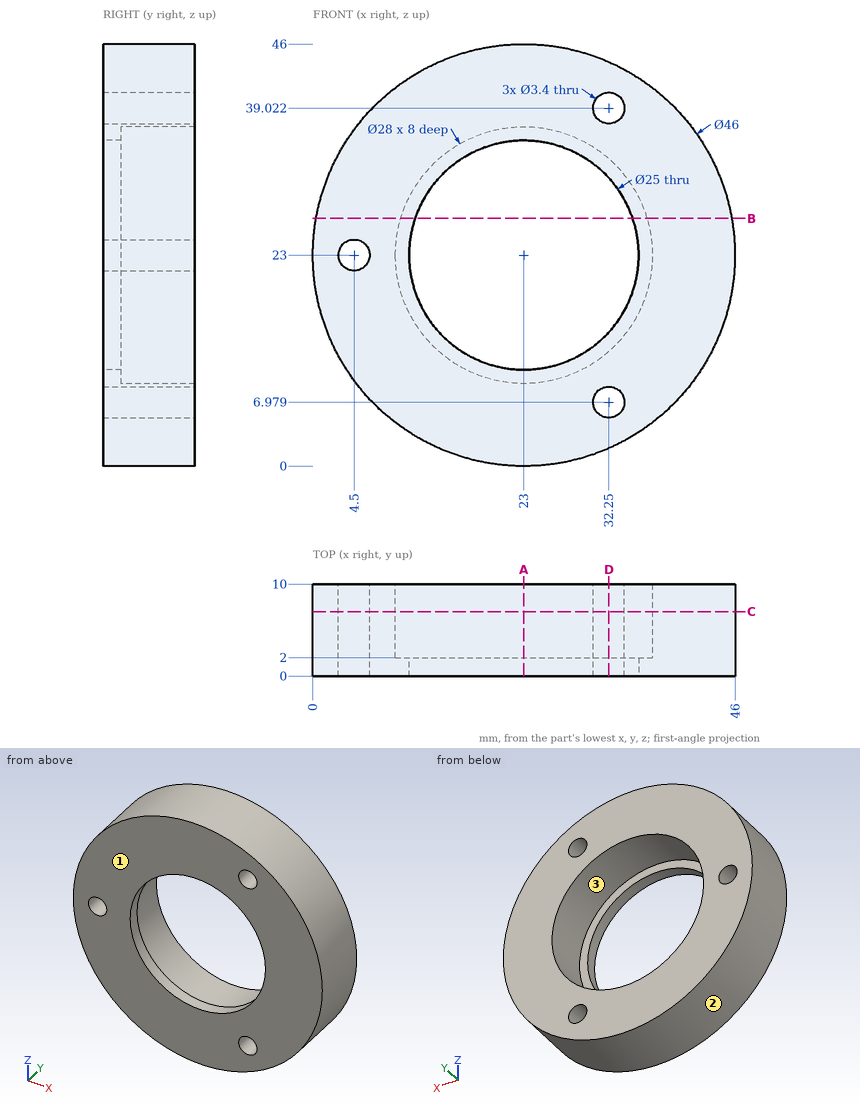
Answer from the drawing. Dimensions are ordinates in mm from the lowest x, y and z of the part. Give positions to 0.01 mm unless a question says otherwise; leave off trailing zeros. Write each loop counter-clockwise with the first axis right and the second up, starting at its lowest first coordinate (ties: lowest second). Pieces come first, ordered by that corner, then holes.
1) For a pull along X with two mould halves and no side action, classify the marked faces 1, 2 and 3 as pulls with the +X half, pulls with the -X half, needs draft (parallel to the pull), parting line crosses it, or undercut.
2) Section C-C (y = 7) is taken. Write down the section's boundary in (x, z).
3) Section B-B (z = 27) is taken. Write down the section's boundary in (x, y).
4) Given P1, Ø1.5, axis at y = 4.5, z = 36.5, coming from the +X side; P2, Ø4, axis at y = 7, z = 10.5, coming from the -X side; P3, Ø2, axis at x = 32.25, z = 6.98, coming from the -Y side; P4, Ø3, axis at y = 4.5, z = 20, coming from the +X side, each flat-ended and moving along its own axis, determine where each tip first touches the part or whether it passes through.
5) Section A-A (x = 23) is taken. Write down the section's boundary in (y, z), and give its area (3 significant figures).
6) Find the intervals of material crossed by L1, parallel to Z at x = 32.25, y = 7; L2, parallel to X at y = 5.25, z = 28.5 (1 decimal); L3, parallel to Z at x = 14.5, y = 3 (1 decimal), in increasing order.
7) Section D-D (x = 32.25) is taken. Write down the section's boundary in (y, z).
Response:
1. face 1: needs draft
1. face 2: parting line crosses it
1. face 3: undercut
2. outline: circle Ø46 at (23, 23); hole circle Ø3.4 at (4.5, 23); hole circle Ø28 at (23, 23); hole circle Ø3.4 at (32.25, 6.98); hole circle Ø3.4 at (32.25, 39.02)
3. outline: (0.35, 0) - (11.16, 0) - (11.16, 2) - (9.58, 2) - (9.58, 10) - (0.35, 10) - close; (34.84, 0) - (45.65, 0) - (45.65, 10) - (36.42, 10) - (36.42, 2) - (34.84, 2) - close
4. P1: stops at x = 42.14
4. P2: stops at x = 2.54
4. P3: passes through
4. P4: stops at x = 45.95
5. outline: (0, 0) - (10, 0) - (10, 9) - (2, 9) - (2, 10.5) - (0, 10.5) - close; (0, 35.5) - (2, 35.5) - (2, 37) - (10, 37) - (10, 46) - (0, 46) - close
5. area: 186 mm2
6. L1: z = 1.94 to 5.28, 8.68 to 12.49, 33.51 to 37.32, 40.72 to 44.06
6. L2: x = 0.7 to 10.1, 35.9 to 45.3
6. L3: z = 1.6 to 11.9, 34.1 to 44.4
7. outline: (0, 1.94) - (10, 1.94) - (10, 5.28) - (0, 5.28) - close; (0, 8.68) - (10, 8.68) - (10, 12.49) - (2, 12.49) - (2, 14.59) - (0, 14.59) - close; (0, 31.41) - (2, 31.41) - (2, 33.51) - (10, 33.51) - (10, 37.32) - (0, 37.32) - close; (0, 40.72) - (10, 40.72) - (10, 44.06) - (0, 44.06) - close
